Work out the finished part from the listing and answer in its coordinate system (mm). Face numbers are marked on the shaded views. A direction names the side the tool comes from. Coordinates: 2 decimals unless noted, no trailing zeros. Order: outer loops, then holes, each group sorted by start corner. A loop starts at its lowest first (then second) coordinate and runs counter-clockwise, first axis right, second up. Notation, with made-up numbers: (72, 69) -> (114, 69) arc R15 ccw to (114, 98) -> close; hole circle Ø9 at (27.25, 63.25). An arc over 180 degrees is marked (long way). Write item = value, one per line. Start each with the question number.
Q1. Which of the six approach directions +Z, -Z, +X, -X, +Y, -Y give full straight-line access (tool end or side, diameter ignored) to the marked faces 5 and 6?
Q2. The part is cut by section C-C, the plane z = -20.5. Count the separate pieces of the cut face and the enclosed holes in it, plus the area to 3 significant figures.
Q3. The part is cut by section B-B, the plane y = 0. Determine the outline of the cut face in (x, z) (3 decimals).
Q4. For a pull along Y with two mould halves and no side action, classify the marked faces 1, 2, 3 and 4 as +Y half, -Y half, draft (parallel to the pull), parting line (faces both ways), or undercut.
Q5. The part is cut by section A-A, the plane x = 0. Determine the outline of the cut face in (y, z) (3 decimals).
Q6. A flat-ended cylindrical pin translates along its axis: pin 1 (1.4 mm diameter, centred on x = -1, z = -37.5, fed in from +Y) (3 decimals). Find the tip coordinate at first contact, or state that the pin passes through.
Q7. Straight lines are drawn through the part: L1, parallel to Y at x = 0, z = -58 (3 decimals); L2, parallel to X at y = -4.5, z = -69; L3, parallel to X at y = 15, z = -16 (3 decimals). For each, find the intervals that lie inside material, in ascending order. Write a range as from..to.
Autodesk Inventor part; units mm, degrees
ref_plane "YZ Plane" through (0, 0, 0) normal (1, 0, 0) x (0, 1, 0)
ref_plane "XZ Plane" through (0, 0, 0) normal (0, 1, 0) x (-1, 0, 0)
ref_plane "XY Plane" through (0, 0, 0) normal (0, 0, 1) x (1, 0, 0)
sketch "Sketch1" plane through (0, 0, 0) normal (0, 0, 1) x (1, 0, 0)
  circle A0 centre (0, 0) radius 3.4
  arc A1 (15.4108, -18.35) -> (15.5882, -17.9217) centre (15.4108, -18.0991) ccw
  line L0 (-15.4108, -18.35) -> (15.4108, -18.35)
  arc A2 (-15.5882, -17.9217) -> (-15.4108, -18.35) centre (-15.4108, -18.0991) ccw
  line L1 (-9.7291, -12.0626) -> (-15.5882, -17.9217)
  arc A3 (-9.1903, -11.8394) -> (-9.7291, -12.0626) centre (-9.1903, -12.6014) ccw
  line L2 (-8.7439, -11.8394) -> (-9.1903, -11.8394)
  arc A4 (-8.7439, -11.8394) -> (-8.2051, -11.6162) centre (-8.7439, -11.0774) ccw
  line L3 (-5.6651, -9.0762) -> (-8.2051, -11.6162)
  arc A5 (-2.3065, -7.685) -> (-5.6651, -9.0762) centre (-2.3065, -12.4348) ccw
  line L4 (2.3065, -7.685) -> (-2.3065, -7.685)
  arc A6 (5.6651, -9.0762) -> (2.3065, -7.685) centre (2.3065, -12.4348) ccw
  line L5 (8.2051, -11.6162) -> (5.6651, -9.0762)
  arc A7 (8.2051, -11.6162) -> (8.7439, -11.8394) centre (8.7439, -11.0774) ccw
  line L6 (9.1903, -11.8394) -> (8.7439, -11.8394)
  arc A8 (9.7291, -12.0626) -> (9.1903, -11.8394) centre (9.1903, -12.6014) ccw
  line L7 (15.5882, -17.9217) -> (9.7291, -12.0626)
  arc A9 (11.7694, -8.6739) -> (11.5462, -8.1351) centre (11.0074, -8.6739) ccw
  line L8 (9.0762, -5.6651) -> (11.5462, -8.1351)
  arc A10 (7.685, -2.3065) -> (9.0762, -5.6651) centre (12.4348, -2.3065) ccw
  line L9 (7.685, 2.3065) -> (7.685, -2.3065)
  arc A11 (9.0762, 5.6651) -> (7.685, 2.3065) centre (12.4348, 2.3065) ccw
  line L10 (11.0322, 7.6211) -> (9.0762, 5.6651)
  arc A12 (11.0322, 7.6211) -> (11.9621, 9.8662) centre (8.7871, 9.8662) ccw
  line L11 (11.9621, 18.5086) -> (11.9621, 9.8662)
  arc A13 (12.3431, 18.8896) -> (11.9621, 18.5086) centre (12.3431, 18.5086) ccw
  line L12 (15.556, 18.8896) -> (12.3431, 18.8896)
  arc A14 (18.35, 16.0956) -> (15.556, 18.8896) centre (15.556, 16.0956) ccw
  line L13 (18.35, -15.3747) -> (18.35, 16.0956)
  arc A15 (17.8962, -15.5627) -> (18.35, -15.3747) centre (18.0841, -15.3747) ccw
  line L14 (11.9926, -9.6591) -> (17.8962, -15.5627)
  arc A16 (11.7694, -9.1203) -> (11.9926, -9.6591) centre (12.5314, -9.1203) ccw
  line L15 (11.7694, -8.6739) -> (11.7694, -9.1203)
  arc A17 (-9.0762, -5.6651) -> (-7.685, -2.3065) centre (-12.4348, -2.3065) ccw
  line L16 (-11.5462, -8.1351) -> (-9.0762, -5.6651)
  arc A18 (-11.5462, -8.1351) -> (-11.7694, -8.6739) centre (-11.0074, -8.6739) ccw
  line L17 (-11.7694, -9.1203) -> (-11.7694, -8.6739)
  arc A19 (-11.9926, -9.6591) -> (-11.7694, -9.1203) centre (-12.5314, -9.1203) ccw
  line L18 (-17.8962, -15.5627) -> (-11.9926, -9.6591)
  arc A20 (-18.35, -15.3747) -> (-17.8962, -15.5627) centre (-18.0841, -15.3747) ccw
  line L19 (-18.35, 16.0956) -> (-18.35, -15.3747)
  arc A21 (-15.556, 18.8896) -> (-18.35, 16.0956) centre (-15.556, 16.0956) ccw
  line L20 (-12.3431, 18.8896) -> (-15.556, 18.8896)
  arc A22 (-11.9621, 18.5086) -> (-12.3431, 18.8896) centre (-12.3431, 18.5086) ccw
  line L21 (-11.9621, 9.8662) -> (-11.9621, 18.5086)
  arc A23 (-11.9621, 9.8662) -> (-11.0322, 7.6211) centre (-8.7871, 9.8662) ccw
  line L22 (-9.0762, 5.6651) -> (-11.0322, 7.6211)
  arc A24 (-7.685, 2.3065) -> (-9.0762, 5.6651) centre (-12.4348, 2.3065) ccw
  line L23 (-7.685, -2.3065) -> (-7.685, 2.3065)
  arc A25 (20, 16.825) -> (16.825, 20) centre (16.825, 16.825) ccw
  line L24 (16.825, 20) -> (5.6287, 20)
  arc A26 (5.6287, 20) -> (4.06, 18.2867) centre (5.6287, 18.4252) ccw
  line L25 (4.06, 18.2867) -> (4.06, 17.5148)
  arc A27 (4.06, 17.5148) -> (5.6348, 15.94) centre (5.6348, 17.5148) ccw
  line L26 (5.6348, 15.94) -> (6.8724, 15.94)
  line L27 (6.8724, 15.94) -> (6.899, 16.702)
  line L28 (6.899, 16.702) -> (9.015, 16.702)
  arc A28 (10.285, 15.432) -> (9.015, 16.702) centre (9.015, 15.432) ccw
  line L29 (10.285, 15.432) -> (10.285, 14.0643)
  arc A29 (10.0246, 13.4357) -> (10.285, 14.0643) centre (9.396, 14.0643) ccw
  line L30 (10.0246, 13.4357) -> (5.6651, 9.0762)
  arc A30 (2.3065, 7.685) -> (5.6651, 9.0762) centre (2.3065, 12.4348) ccw
  line L31 (2.3065, 7.685) -> (-2.3065, 7.685)
  arc A31 (-5.6651, 9.0762) -> (-2.3065, 7.685) centre (-2.3065, 12.4348) ccw
  line L32 (-5.6651, 9.0762) -> (-10.0246, 13.4357)
  arc A32 (-10.285, 14.0643) -> (-10.0246, 13.4357) centre (-9.396, 14.0643) ccw
  line L33 (-10.285, 14.0643) -> (-10.285, 15.432)
  arc A33 (-9.015, 16.702) -> (-10.285, 15.432) centre (-9.015, 15.432) ccw
  line L34 (-9.015, 16.702) -> (-6.899, 16.702)
  line L35 (-6.899, 16.702) -> (-6.8724, 15.94)
  line L36 (-6.8724, 15.94) -> (-5.6348, 15.94)
  arc A34 (-5.6348, 15.94) -> (-4.06, 17.5148) centre (-5.6348, 17.5148) ccw
  line L37 (-4.06, 17.5148) -> (-4.06, 18.2867)
  arc A35 (-4.06, 18.2867) -> (-5.6287, 20) centre (-5.6287, 18.4252) ccw
  line L38 (-5.6287, 20) -> (-16.825, 20)
  arc A36 (-16.825, 20) -> (-20, 16.825) centre (-16.825, 16.825) ccw
  line L39 (-20, 16.825) -> (-20, -16.825)
  arc A37 (-20, -16.825) -> (-16.825, -20) centre (-16.825, -16.825) ccw
  line L40 (-16.825, -20) -> (16.825, -20)
  arc A38 (16.825, -20) -> (20, -16.825) centre (16.825, -16.825) ccw
  line L41 (20, -16.825) -> (20, 16.825)
extrude "Extrusion1" add sketch "Sketch1" against normal blind 100
properties part number "40-4001-BLACK-FB"
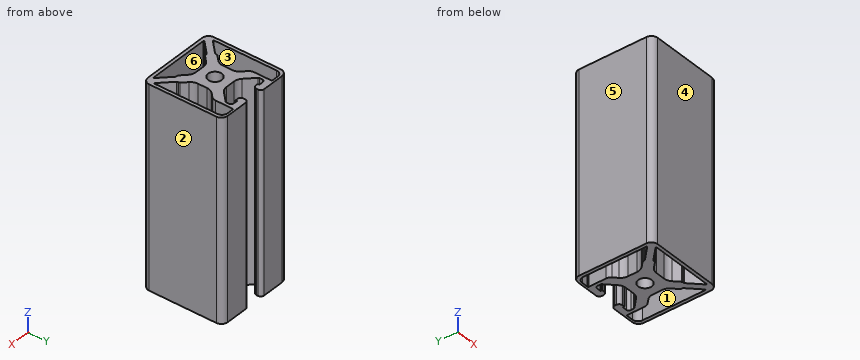
Model answer:
q1.face_5 = +Z, -Z, -X, +Y, -Y
q1.face_6 = +Z, -Z
q2.separate_pieces = 1
q2.enclosed_holes = 4
q2.area = 655 mm2
q3.outline = (-20, -100) -> (-18.35, -100) -> (-18.35, 0) -> (-20, 0) -> close; (-7.685, -100) -> (-3.4, -100) -> (-3.4, 0) -> (-7.685, 0) -> close; (3.4, -100) -> (7.685, -100) -> (7.685, 0) -> (3.4, 0) -> close; (18.35, -100) -> (20, -100) -> (20, 0) -> (18.35, 0) -> close
q4.face_1 = undercut
q4.face_2 = draft
q4.face_3 = undercut
q4.face_4 = -Y half
q5.outline = (-20, -100) -> (-18.35, -100) -> (-18.35, 0) -> (-20, 0) -> close; (-7.685, -100) -> (-3.4, -100) -> (-3.4, 0) -> (-7.685, 0) -> close; (3.4, -100) -> (7.685, -100) -> (7.685, 0) -> (3.4, 0) -> close
q6.pin_1 = 7.685
q7.L1 = -20..-18.35, -7.685..-3.4, 3.4..7.685
q7.L2 = -20..-18.35, -8.22..8.22, 18.35..20
q7.L3 = -20..-18.35, -11.962..-10.285, 10.285..11.962, 18.35..20
